Geometry: final body of the model. Coordinates: model frame, mm. A direction names the side the tool comes from. Give positions to 0.01 mm unless a question says otherwise; leave off trailing zeros. Loops run counter-clockwise (first coordinate to the right, second up) from the corner with the lowest first, then second, coordinate; pieces in that order, holes last.
1. Access query for faces 4 (the face through (-1.217, 24.014, -17.837)), 5 (the face through (0, 12, -35.5)), 6 (the face through (16.882, 1.014, -23.682)), 7 (the face through (0, 34, 8)). Directions: +Z, -Z, +X, -X, +Y, -Y. A direction counts if a zero-diameter tool reaches every point of the face in a straight line with its end or side. Return the directions, or none.
2. Section A-A, the plane z = 16.25. Output: boundary loops of the cut face in (x, y).
3. Section B-B, the plane y = 27.5. Output: boundary loops of the cut face in (x, z), then the cut area to 3 significant figures.
4. First-contact query: P1, Ø3, axis at x = 0.5, y = 31, coming from the -Z side; P2, Ø1.6, axis at x = 29, y = 24, coming from the +Z side; P3, Ø1.8, axis at y = 28.5, z = 27, coming from the +X side; P4, Ø2.5, axis at x = -23.72, z = -10.28, coming from the +Y side. Flat tips, straight axial feed; report the tip coordinate or a pass-through.
5. Material intervals for line 1 along X through (y, z) = (24.5, 6); line 2 along Y through (x, z) = (-1, -25); line 3 along Y through (x, z) = (-36.05, 16.25), sorted ascending.
6. Section C-C, the plane x = 26.5. Output: boundary loops of the cut face in (y, z).
7. Section D-D, the plane z = 26. Output: boundary loops of the cut face in (x, y), then the cut area to 3 significant figures.
8. Draft query along Y for faces 1 (the face through (26, 1, -22.118)), 2 (the face through (0, 29, 28)), 3 (the face through (-37, 15, 22)). Return one class per face: +Y half, -Y half, draft (parallel to the pull), parting line (faces both ways), or undercut.
from build123d import *

# Parameters (mm, degrees)
SKETCH2_W           = 75
SKETCH2_H           = 75
BOSS_EXTRUDE1_DEPTH = 25
SHELL1_T            = -2
SKETCH3_R           = 1.6
CUT_EXTRUDE1_DEPTH  = 50
CUT_EXTRUDE2_DEPTH  = 10
BOSS_EXTRUDE2_START = -5
BOSS_EXTRUDE2_DEPTH = 10
LPATTERN1_COUNT     = 2
LPATTERN1_PITCH     = 20
SKETCH7_R           = 1.6
CUT_EXTRUDE4_DEPTH  = 10
SKETCH9_R           = 1.6
CUT_EXTRUDE5_DEPTH  = 10
SKETCH10_R          = 2
CUT_EXTRUDE6_DEPTH  = 10
CUT_EXTRUDE7_START  = -10
CUT_EXTRUDE7_DEPTH  = 10


with BuildPart() as part:
    # Sketch2 → Boss-Extrude1 (new body)
    with BuildSketch(Plane(origin=(0, 0, 0), x_dir=(1, 0, 0), z_dir=(0, 1, 0))):
        Rectangle(SKETCH2_W, SKETCH2_H)
    extrude(amount=BOSS_EXTRUDE1_DEPTH)

    # Shell1
    shell1_openings = [part.faces().sort_by_distance(p)[0] for p in [
        (0, 12.5, 37.5),
        (37.5, 12.5, 0),
    ]]
    offset(amount=SHELL1_T, openings=shell1_openings, kind=Kind.INTERSECTION)

    # Sketch3 → Cut-Extrude1 (cut)
    with BuildSketch(Plane(origin=(0, 2, 0), x_dir=(1, 0, 0), z_dir=(0, 1, 0))):
        with Locations(Location((-23.717514421, 23.717514421, 0), (0, 0, 270))):
            Circle(SKETCH3_R)
        with Locations(Location((-10.282485579, 23.717514421, 0), (0, 0, 270))):
            Circle(SKETCH3_R)
        with Locations(Location((-10.282485579, 10.282485579, 0), (0, 0, 270))):
            Circle(SKETCH3_R)
        with Locations(Location((-23.717514421, 10.282485579, 0), (0, 0, 270))):
            Circle(SKETCH3_R)
        with Locations(Location((10.282485579, 23.717514421, 0), (0, 0, 270))):
            Circle(SKETCH3_R)
        with Locations(Location((23.717514421, 23.717514421, 0), (0, 0, 270))):
            Circle(SKETCH3_R)
        with Locations(Location((10.282485579, 10.282485579, 0), (0, 0, 270))):
            Circle(SKETCH3_R)
        with Locations(Location((23.717514421, 10.282485579, 0), (0, 0, 270))):
            Circle(SKETCH3_R)
    extrude(amount=-CUT_EXTRUDE1_DEPTH, mode=Mode.SUBTRACT)

    # Sketch4 → Cut-Extrude2 (cut)
    with BuildSketch(Plane(origin=(0, 25, 0), x_dir=(1, 0, 0), z_dir=(0, 1, 0))):
        with BuildLine():
            Line((-37.5, -37.5), (-13.25, -37.5))
            Line((-13.25, -37.5), (-13.25, -7.5))
            Line((-13.25, -7.5), (-13.25, 17))
            ThreePointArc((-13.25, 17), (-17, 20.75), (-20.75, 17))
            Line((-20.75, 17), (-20.75, -7.5))
            Line((-20.75, -7.5), (-37.5, -7.5))
            Line((-37.5, -7.5), (-37.5, -37.5))
        make_face()
        with BuildLine():
            Line((37.5, -37.5), (37.5, -7.5))
            Line((37.5, -7.5), (20.75, -7.5))
            Line((20.75, -7.5), (20.75, 17))
            ThreePointArc((20.75, 17), (17, 20.75), (13.25, 17))
            Line((13.25, 17), (13.25, -7.5))
            Line((13.25, -7.5), (13.25, -37.5))
            Line((13.25, -37.5), (37.5, -37.5))
        make_face()
    extrude(amount=-CUT_EXTRUDE2_DEPTH, mode=Mode.SUBTRACT)

    # Sketch5 → Boss-Extrude2 (add)
    with BuildSketch(Plane.XY.offset(37.5).offset(BOSS_EXTRUDE2_START)):
        with BuildLine():
            Line((-5, 25), (-5, 31))
            ThreePointArc((-5, 31), (0, 36), (5, 31))
            Line((5, 31), (5, 25))
            Line((5, 25), (-5, 25))
        make_face()
        with BuildLine():
            Line((-3, 31), (-3, 29))
            Line((-3, 29), (3, 29))
            Line((3, 29), (3, 31))
            ThreePointArc((3, 31), (0, 34), (-3, 31))
        make_face(mode=Mode.SUBTRACT)
    boss_extrude2 = extrude(amount=-BOSS_EXTRUDE2_DEPTH)

    # LPattern1: Boss-Extrude2 ×2
    with Locations(*[(0, 0, -i * LPATTERN1_PITCH) for i in range(1, LPATTERN1_COUNT)]):
        add(boss_extrude2)

    # Sketch7 → Cut-Extrude4 (cut)
    with BuildSketch(Plane.XZ):
        with Locations(Location((0, 16.25, 0), (0, 0, 270))):
            Circle(SKETCH7_R)
        with Locations(Location((16.25, 0, 0), (0, 0, 270))):
            Circle(SKETCH7_R)
        with Locations(Location((0, -16.25, 0), (0, 0, 270))):
            Circle(SKETCH7_R)
        with Locations(Location((-16.25, 0, 0), (0, 0, 270))):
            Circle(SKETCH7_R)
    extrude(amount=-CUT_EXTRUDE4_DEPTH, mode=Mode.SUBTRACT)

    # Sketch9 → Cut-Extrude5 (cut)
    with BuildSketch(Plane(origin=(-35.5, 0, 0), x_dir=(0, 0, -1), z_dir=(1, 0, 0))):
        with Locations((-16.25, 8)):
            Circle(SKETCH9_R)
        with Locations((16.25, 8)):
            Circle(SKETCH9_R)
    extrude(amount=-CUT_EXTRUDE5_DEPTH, mode=Mode.SUBTRACT)

    # Sketch10 → Cut-Extrude6 (cut)
    with BuildSketch(Plane(origin=(0, 25, 0), x_dir=(1, 0, 0), z_dir=(0, 1, 0))):
        with Locations(Location((0, 16.25, 0), (0, 0, 270))):
            Circle(SKETCH10_R)
    extrude(amount=-CUT_EXTRUDE6_DEPTH, mode=Mode.SUBTRACT)

    # Sketch11 → Cut-Extrude7 (cut)
    with BuildSketch(Plane.XZ.offset(CUT_EXTRUDE7_START)):
        with BuildLine():
            Line((10.282485579, -8.682485579), (15.282485579, -8.682485579))
            ThreePointArc((15.282485579, -8.682485579), (16.882485579, -10.282485579), (15.282485579, -11.882485579))
            Line((15.282485579, -11.882485579), (10.282485579, -11.882485579))
            ThreePointArc((10.282485579, -11.882485579), (8.682485579, -10.282485579), (10.282485579, -8.682485579))
        make_face()
        with BuildLine():
            Line((23.717514421, -8.682485579), (28.717514421, -8.682485579))
            ThreePointArc((28.717514421, -8.682485579), (30.317514421, -10.282485579), (28.717514421, -11.882485579))
            Line((28.717514421, -11.882485579), (23.717514421, -11.882485579))
            ThreePointArc((23.717514421, -11.882485579), (22.117514421, -10.282485579), (23.717514421, -8.682485579))
        make_face()
        with BuildLine():
            Line((23.717514421, -22.117514421), (28.717514421, -22.117514421))
            ThreePointArc((28.717514421, -22.117514421), (30.317514421, -23.717514421), (28.717514421, -25.317514421))
            Line((28.717514421, -25.317514421), (23.717514421, -25.317514421))
            ThreePointArc((23.717514421, -25.317514421), (22.117514421, -23.717514421), (23.717514421, -22.117514421))
        make_face()
        with BuildLine():
            Line((10.282485579, -22.117514421), (15.282485579, -22.117514421))
            ThreePointArc((15.282485579, -22.117514421), (16.882485579, -23.717514421), (15.282485579, -25.317514421))
            Line((15.282485579, -25.317514421), (10.282485579, -25.317514421))
            ThreePointArc((10.282485579, -25.317514421), (8.682485579, -23.717514421), (10.282485579, -22.117514421))
        make_face()
    extrude(amount=CUT_EXTRUDE7_DEPTH, mode=Mode.SUBTRACT)


solid = part.part
Answers below:
1. face 4: +Y
1. face 5: +Z, +X
1. face 6: -Y
1. face 7: +Z, -Z
2. outline: (-37.5, 0) - (-1.6, 0) - (-1.6, 2) - (-35.5, 2) - (-35.5, 6.4) - (-37.5, 6.4) - close; (-37.5, 9.6) - (-35.5, 9.6) - (-35.5, 15) - (-37.5, 15) - close; (-13.25, 23) - (13.25, 23) - (13.25, 25) - (-13.25, 25) - close; (1.6, 0) - (37.5, 0) - (37.5, 2) - (1.6, 2) - close
3. outline: (-5, 2.5) - (5, 2.5) - (5, 12.5) - (-5, 12.5) - close; (-5, 22.5) - (5, 22.5) - (5, 32.5) - (-5, 32.5) - close
3. area: 200 mm2
4. P1: passes through
4. P2: stops at z = 7.5
4. P3: stops at x = 5
4. P4: stops at y = 25
5. line 1: x = -37.5 to -20.75, -13.25 to 13.25, 20.75 to 37.5
5. line 2: y = 0 to 2, 23 to 25
5. line 3: y = 0 to 6.4, 9.6 to 15
6. outline: (0, -37.5) - (25, -37.5) - (25, 7.5) - (23, 7.5) - (23, -35.5) - (2, -35.5) - (2, -25.32) - (0, -25.32) - close; (0, -22.12) - (2, -22.12) - (2, -11.88) - (0, -11.88) - close; (0, -8.68) - (2, -8.68) - (2, 37.5) - (0, 37.5) - close
7. outline: (-37.5, 0) - (37.5, 0) - (37.5, 2) - (-35.5, 2) - (-35.5, 15) - (-37.5, 15) - close; (-13.25, 23) - (13.25, 23) - (13.25, 25) - (5, 25) - (5, 31) arc R5 ccw to (-5, 31) - (-5, 25) - (-13.25, 25) - close; hole (-3, 29) - (3, 29) - (3, 31) arc R3 ccw to (-3, 31) - close
7. area: 302 mm2
8. face 1: draft
8. face 2: undercut
8. face 3: +Y half
